Job drawing, mm, ordinate dimensions from the low corner. One solid piece. A direction names the side the tool comes from. Give positions to 0.01 mm unless a question says otherwise; leave off trailing zeros. Loops run counter-clockwise (first coordinate to the right, second up) from the corner with the lowest first, then second, coordinate; pieces in that order, holes last. Notation, with made-up numbers: (-39, 18) -> (3, 18) arc R10 cw to (3, 25) -> close; hole circle Ø11 at (-39, 53). An arc over 180 degrees is marked (long way). Use one line per item in the form item = value.
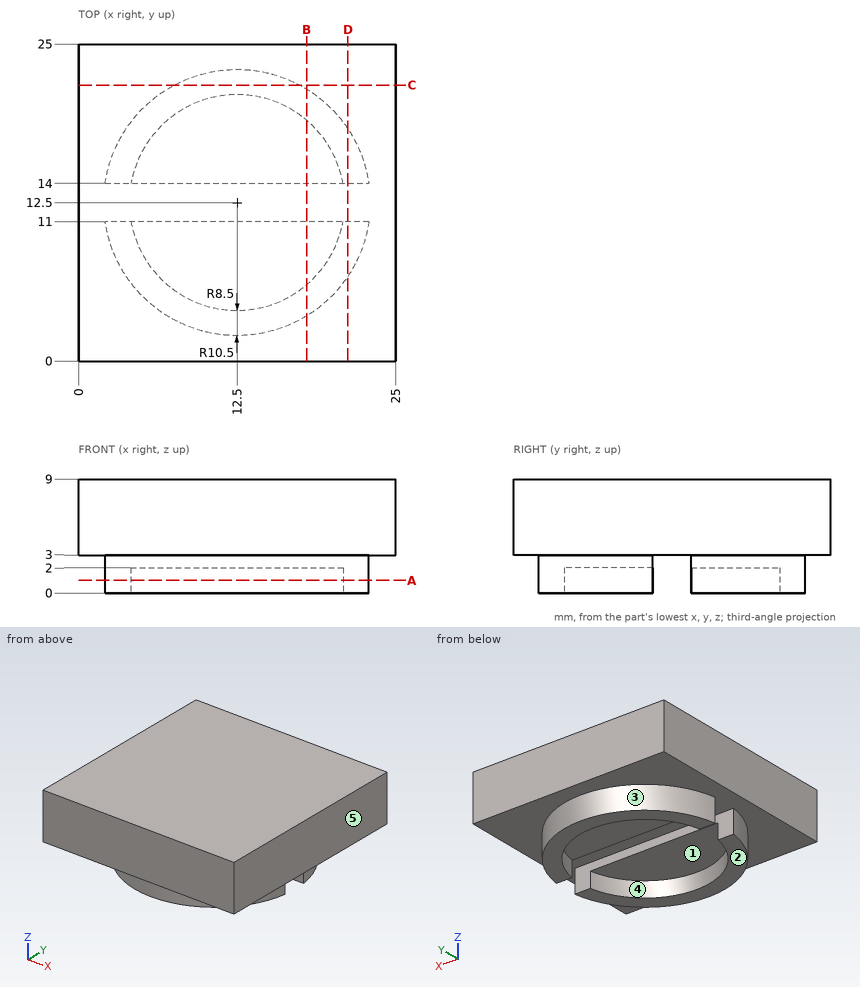
1. Cut at B-B, the plane x = 18. Write the cut outline in (y, z), then the cut area to 3 significant figures.
Result sheet:
outline = (0, 3) -> (3.56, 3) -> (3.56, 0) -> (6.02, 0) -> (6.02, 2) -> (11, 2) -> (11, 3) -> (14, 3) -> (14, 2) -> (18.98, 2) -> (18.98, 0) -> (21.44, 0) -> (21.44, 3) -> (25, 3) -> (25, 9) -> (0, 9) -> close
area = 175 mm^2
2. Tool access for the marked faces 4 and 5: list every direction of +Z, -Z, +X, -X, +Y, -Y with a clear straight run to the whole face (end or side of a thin tool).
Result sheet:
face_4 = -Z
face_5 = +Z, -Z, +X, +Y, -Y
3. Cut at C-C, the plane y = 21.75. Write the cut outline in (x, z).
Result sheet:
outline = (0, 3) -> (7.53, 3) -> (7.53, 0) -> (17.47, 0) -> (17.47, 3) -> (25, 3) -> (25, 9) -> (0, 9) -> close
4. Drop flat-ended pins along their axis: P1, Ø1, axis at x = 8, z = 4, coming from the -Y side; P2, Ø3, axis at y = 21.5, z = 1, coming from the -X side; P3, Ø1.5, axis at x = 12.5, z = 1, coming from the -Y side; P4, Ø2, axis at x = 7, z = 1, coming from the -Y side. Give the stop position or say it passes through.
Result sheet:
P1 = 0
P2 = 5.15
P3 = 2
P4 = 3.01
5. Mould opens along Y. For the marked faces 1, 2 and 3 say: pulls with the +Y half, pulls with the -Y half, needs draft (parallel to the pull), parting line crosses it, or undercut.
Result sheet:
face_1 = undercut
face_2 = needs draft
face_3 = pulls with the +Y half
6. Drill centre lines: line 1 (Z direction, x = 2.5, y = 1.75); line 2 (X direction, y = 19.5, z = 1.5); line 3 (X direction, y = 20.25, z = 1.5). Where is each one in solid material? Low to high.
Result sheet:
line_1 = 3 to 9
line_2 = 4.67 to 7.68, 17.32 to 20.33
line_3 = 5.42 to 9.01, 15.99 to 19.58
7. Cut at A-A, the plane z = 1. Write the cut outline in (x, y).
Result sheet:
outline = (2.11, 11) arc R10.5 ccw to (22.89, 11) -> (20.87, 11) arc R8.5 cw to (4.13, 11) -> close; (2.11, 14) -> (4.13, 14) arc R8.5 cw to (20.87, 14) -> (22.89, 14) arc R10.5 ccw to start
8. Cut at D-D, the plane x = 21.25. Write the cut outline in (y, z).
Result sheet:
outline = (0, 3) -> (6.7, 3) -> (6.7, 0) -> (11, 0) -> (11, 3) -> (14, 3) -> (14, 0) -> (18.3, 0) -> (18.3, 3) -> (25, 3) -> (25, 9) -> (0, 9) -> close
